Work out the finished part from the listing and answer in its coordinate system (mm). Face numbers are marked on the shaded views. A direction names the side the tool comes from. Give positions to 0.01 mm unless a question says otherwise; leave off trailing zeros. Loops run counter-clockwise (first coordinate to the right, second up) from the corner with the lowest first, then second, coordinate; pieces in that order, holes last. Notation, with made-up numbers: M -14,79 L 2,79 A20 cw 2,110 Z; hole C 50,-21 d5. An arc over 180 degrees is marked long. Use a Markdown table: item, result.
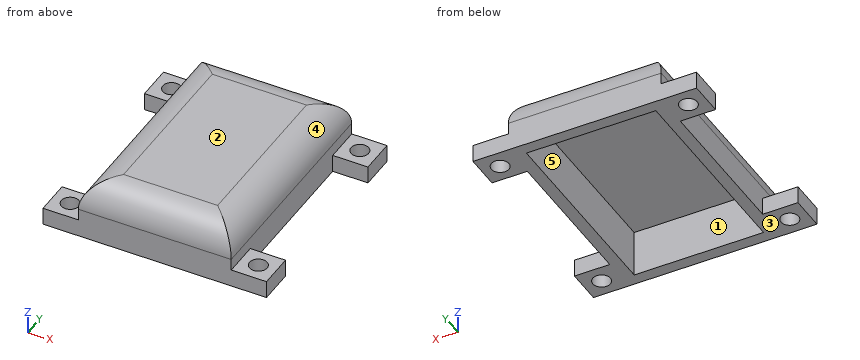
```python
from build123d import *

# Parameters (mm, degrees)
SKETCH_1_W          = 26
SKETCH_1_H          = 38
EXTRUDE_1_DEPTH     = 10
SKETCH_2_W          = 22
SKETCH_2_H          = 34
CUT_EXTRUDE_1_DEPTH = 8
SKETCH_4_W          = 6
SKETCH_4_H          = 6
EXTRUDE_2_DEPTH     = 3
SKETCH_5_R          = 1.5
CUT_EXTRUDE_4_DEPTH = 11
FILLET_1_R          = 5


with BuildPart() as part:
    # ｽｹｯﾁ1 → ﾎﾞｽ - 押し出し1 (new body)
    with BuildSketch(Plane.XY):
        Rectangle(SKETCH_1_W, SKETCH_1_H)
    extrude(amount=EXTRUDE_1_DEPTH)

    # ｽｹｯﾁ2 → ｶｯﾄ - 押し出し1 (cut)
    with BuildSketch(Plane.XY):
        Rectangle(SKETCH_2_W, SKETCH_2_H)
    extrude(amount=CUT_EXTRUDE_1_DEPTH, mode=Mode.SUBTRACT)

    # ｽｹｯﾁ4 → ﾎﾞｽ - 押し出し2 (add)
    with BuildSketch(Plane.XY):
        with Locations((16, 16)):
            Rectangle(SKETCH_4_W, SKETCH_4_H)
        with Locations((16, -16)):
            Rectangle(SKETCH_4_W, SKETCH_4_H)
        with Locations((-16, -16)):
            Rectangle(SKETCH_4_W, SKETCH_4_H)
        with Locations((-16, 16)):
            Rectangle(SKETCH_4_W, SKETCH_4_H)
    extrude(amount=EXTRUDE_2_DEPTH)

    # ｽｹｯﾁ5 → ｶｯﾄ - 押し出し4 (cut, through all)
    with BuildSketch(Plane.XY):
        with Locations((-16, 16)):
            Circle(SKETCH_5_R)
        with Locations((-16, -16)):
            Circle(SKETCH_5_R)
        with Locations((16, -16)):
            Circle(SKETCH_5_R)
        with Locations((16, 16)):
            Circle(SKETCH_5_R)
    extrude(amount=CUT_EXTRUDE_4_DEPTH, mode=Mode.SUBTRACT)

    # ﾌｨﾚｯﾄ1
    fillet_1_edges = [part.edges().sort_by_distance(p)[0] for p in [
        (0, 19, 10),
        (0, -19, 10),
        (13, 0, 10),
        (-13, 0, 10),
    ]]
    fillet(fillet_1_edges, radius=FILLET_1_R)


solid = part.part
```
(1) A cutting plane is placed at D-D (x = 4). Write down the section's boundary in (y, z).
Entries:
| item | result |
|---|---|
| outline | M -19,0 L -17,0 L -17,8 L 17,8 L 17,0 L 19,0 L 19,5 A5 ccw 14,10 L -14,10 A5 ccw -19,5 Z |
(2) A cutting plane is placed at B-B (y = 16). Write down the section's boundary in (x, z), and give its area (3 significant figures).
Entries:
| item | result |
|---|---|
| outline | M -19,0 L -17.5,0 L -17.5,3 L -19,3 Z; M -14.5,0 L -11,0 L -11,8 L 11,8 L 11,0 L 14.5,0 L 14.5,3 L 13,3 L 13,5 A5 ccw 10,9.58 L -10,9.58 A5 ccw -13,5 L -13,3 L -14.5,3 Z; M 17.5,0 L 19,0 L 19,3 L 17.5,3 Z |
| area | 83.5 mm² |
(3) A cutting plane is placed at C-C (z = 6.5). Write down the section's boundary in (x, y).
Entries:
| item | result |
|---|---|
| outline | M -12.77,-18.77 L 12.77,-18.77 L 12.77,18.77 L -12.77,18.77 Z; hole M -11,-17 L 11,-17 L 11,17 L -11,17 Z |
(4) A cutting plane is placed at A-A (x = 16). Write down the section's boundary in (y, z), and give its area (3 significant figures).
Entries:
| item | result |
|---|---|
| outline | M -19,0 L -17.5,0 L -17.5,3 L -19,3 Z; M -14.5,0 L -13,0 L -13,3 L -14.5,3 Z; M 13,0 L 14.5,0 L 14.5,3 L 13,3 Z; M 17.5,0 L 19,0 L 19,3 L 17.5,3 Z |
| area | 18.0 mm² |
(5) The mould has two halves that part along X. Classify the marked faces 3, 4 and 5: released by +X, released by -X, zero draft, split by the parting line, or undercut.
Entries:
| item | result |
|---|---|
| face 3 | zero draft |
| face 4 | released by +X |
| face 5 | undercut |
(6) Which of the six approach directions +Z, -Z, +X, -X, +Y, -Y give full straight-line access (tool end or side, diameter ignored) to the marked faces 1 and 2?
Entries:
| item | result |
|---|---|
| face 1 | -Z |
| face 2 | +Z, +X, -X, +Y, -Y |
(7) Consider probe 1 along X at (y, z) = (16, 0.7); probe 2 along Y at (x, z) = (-10.5, 3.5); probe 3 along X at (y, z) = (1.5, 4.5). Determine where each line is inside the solid, lowest interval first. Write a range as [from, to].
Entries:
| item | result |
|---|---|
| probe 1 | x = [-19, -17.5], [-14.5, -11], [11, 14.5], [17.5, 19] |
| probe 2 | y = [-19, -17], [17, 19] |
| probe 3 | x = [-13, -11], [11, 13] |
(8) Given P1, Ø12, axis at x = 10.5, y = 10.5, coming from the -Z side; P2, Ø1, axis at y = 7.5, z = 5, coming from the -X side; P3, Ø1.8, axis at x = -16, y = 15, coming from the +Z side, each flat-ended and moving along its own axis, determine where each tip first touches the part or whether it passes through.
Entries:
| item | result |
|---|---|
| P1 | stops at z = 0 |
| P2 | stops at x = -13 |
| P3 | stops at z = 3 |
